```python
from build123d import *

# Parameters (mm, degrees)
EXTRUDE_1_DEPTH = 20
EXTRUDE_4_DEPTH = 20
SKETCH_10_R     = 6
EXTRUDE_5_DEPTH = 4


with BuildPart() as part:
    # 草图2 → 凸台-拉伸1 (new body, symmetric)
    with BuildSketch(Plane(origin=(0, 0, 0), x_dir=(0, 0, -1), z_dir=(1, 0, 0))):
        Polygon((-10, 1), (-8, 1), (-8, -1), (-10, -1), (-12, -1), (-12, 1), align=None)
    extrude(amount=EXTRUDE_1_DEPTH, both=True)

    # 草图9 → 凸台-拉伸4 (add)
    with BuildSketch(Plane(origin=(0, 1, 0), x_dir=(1, 0, 0), z_dir=(0, 1, 0))):
        with BuildLine():
            Line((-40, -8), (40, -8))
            ThreePointArc((40, -8), (99.39696962, -32.60303038), (124, -92))
            Line((124, -92), (124, -108))
            Line((124, -108), (120, -108))
            Line((120, -108), (120, -92))
            ThreePointArc((120, -92), (96.568542495, -35.431457505), (40, -12))
            Line((40, -12), (-40, -12))
            ThreePointArc((-40, -12), (-96.568542495, -35.431457505), (-120, -92))
            Line((-120, -92), (-120, -108))
            Line((-120, -108), (-124, -108))
            Line((-124, -108), (-124, -92))
            ThreePointArc((-124, -92), (-99.39696962, -32.60303038), (-40, -8))
        make_face()
    extrude(amount=EXTRUDE_4_DEPTH)

    # 草图10 → 凸台-拉伸5 (add)
    with BuildSketch(Plane(origin=(0, 0, 8), x_dir=(-1, 0, 0), z_dir=(0, 0, -1))):
        with Locations((0, 11)):
            Circle(SKETCH_10_R)
    extrude(amount=EXTRUDE_5_DEPTH)


solid = part.part
```
Could you check a few things on this model? Use its own coordinates, in mm. A direction names the side the tool comes from. Coordinates: 2 decimals unless noted, no trailing zeros. Loops run counter-clockwise (first coordinate to the right, second up) from the corner with the lowest first, then second, coordinate; pieces in that order, holes last.
1) Imagine slicing it at C-C (y = 11). List the corners of the cut face in (x, z) for me, and give its area (3 significant figures).
Reported:
outline: (-124, 92) arc R84 ccw to (-40, 8) - (-6, 8) - (-6, 4) - (6, 4) - (6, 8) - (40, 8) arc R84 ccw to (124, 92) - (124, 108) - (120, 108) - (120, 92) arc R80 cw to (40, 12) - (-40, 12) arc R80 cw to (-120, 92) - (-120, 108) - (-124, 108) - close
area: 1,530 mm2
2) Imagine slicing it at D-D (z = 48.5). List the corners of the cut face in (x, y) for me.
Reported:
outline: (-111.86, 1) - (-107.14, 1) - (-107.14, 21) - (-111.86, 21) - close; (107.14, 1) - (111.86, 1) - (111.86, 21) - (107.14, 21) - close
3) Imagine slicing it at B-B (x = 0). List the corners of the cut face in (y, z) for me, and give its area (3 significant figures).
Reported:
outline: (-1, 8) - (5, 8) - (5, 4) - (17, 4) - (17, 8) - (21, 8) - (21, 12) - (-1, 12) - close
area: 136 mm2
4) Which directions (+Z, -Z, +X, -X, +Y, -Y) give clear straight access to the entire face, cutting with the end or side of a thin tool? Please do faces 1 (the face through (-124, 11, 100)), 2 (the face through (97.19, 10.86, 36.06)), 3 (the face through (95, 1, 32)), 4 (the face through (1.301, 5.143, 6.028)).
Reported:
face 1: +Z, -Z, -X, +Y, -Y
face 2: +Z, +Y, -Y
face 3: +Z, -Z, +X, -Y
face 4: -Z
5) Will these pins go through, and if not, where does the flat tip stop? pin 1 Ø11 at (x, y) = (-9.5, 9.5) entering from -Z; pin 2 Ø6 at (x, y) = (-14, 5) entering from +Z; pin 3 Ø0.6 at (y, z) = (0, 9) entering from -X; pin 4 Ø4 at (x, y) = (77.5, 12.5) entering from +Z.
Reported:
pin 1: stops at z = 4
pin 2: stops at z = 12
pin 3: stops at x = -20
pin 4: stops at z = 22.43
6) Imagine slicing it at A-A (z = 31). List the corners of the cut face in (x, y) for me, and give its area (3 significant figures).
Reported:
outline: (-97.75, 1) - (-91.76, 1) - (-91.76, 21) - (-97.75, 21) - close; (91.76, 1) - (97.75, 1) - (97.75, 21) - (91.76, 21) - close
area: 240 mm2
7) Thinking about a two-plate mould opening in X: for faces 5 (the face through (-95, 1, 32)), 6 (the face through (-120, 11, 100)), 7 (the face through (98.74, 10.86, 31.954)), which applies, released by +X, released by -X, zero draft, split by the parting line, or undercut?
Reported:
face 5: zero draft
face 6: undercut
face 7: released by +X
8) Please list where these lines run through material, in increasing order: line 1 along X through (y, z) = (3, 94.5); line 2 along X through (y, z) = (16.5, 55.5); line 3 along Z through (x, y) = (-105, 14.75).
Reported:
line 1: x = -124 to -120, 120 to 124
line 2: x = -115.66 to -111.19, 111.19 to 115.66
line 3: z = 38.79 to 45.36
